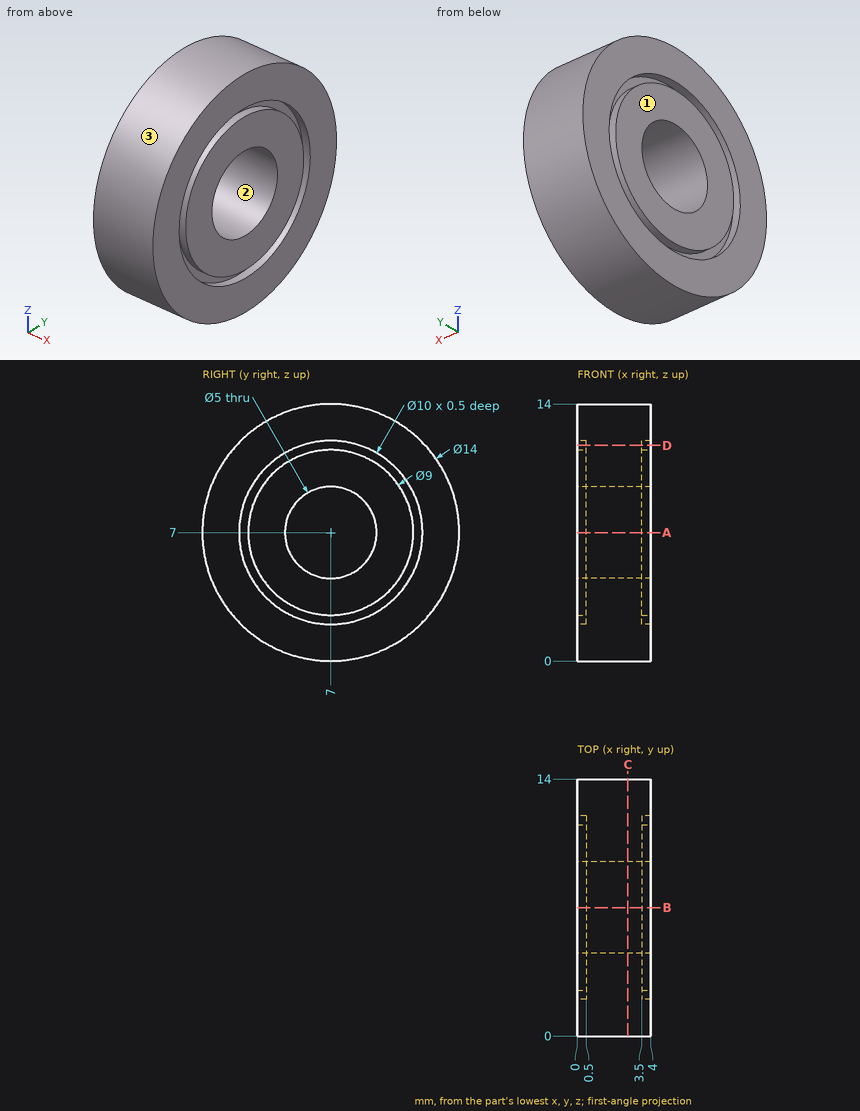
For this review, use the dimensioned drawing (mm, ordinates from the lowest corner) and the shaded views. Round coordinates to 2 decimals unless told otherwise and drop trailing zeros. Order: outer loops, then holes, each group sorted by start corner. A loop starts at its lowest first (then second) coordinate and runs counter-clockwise, first axis right, second up. Notation, with made-up numbers: (39, 10.5) -> (90, 10.5) arc R34 ccw to (90, 41.5) -> close; hole circle Ø4 at (62, 7.25). An arc over 180 degrees is marked (long way). One line per item, written item: value. Start each with the question number.
Q1. Clearance check with flat-ended pins moving along their axes: pin 1 Ø1 at (x, z) = (2, 3.5) entering from -Y; pin 2 Ø1 at (x, y) = (3, 12.5) entering from +Z. State where each tip first meets the part, or that it passes through.
Q2. Mouldability with a two-part tool opening along Z and no side actions: class the marked faces 1, 2 and 3 as released by +Z, released by -Z, zero draft, split by the parting line, or undercut.
Q3. Take a section at D-D (z = 11.75). Write out the cut boundary in (x, y), and give its area (3 significant figures).
Q4. Take a section at A-A (z = 7). Write out the cut boundary in (x, y).
Q5. Wall thickness on line 1 (Y direction, x = 3.65, z = 7); line 2 (Y direction, x = 3.55, z = 5.25); line 3 (Y direction, x = 0.6, z = 5): over which ranges is each line inside the solid? List them lowest first.
Q6. Take a section at C-C (x = 2.75). Write out the cut boundary in (y, z).
Reported:
1. pin 1: stops at y = 0.68
1. pin 2: stops at z = 11.9
2. face 1: zero draft
2. face 2: undercut
2. face 3: split by the parting line
3. outline: (0, 1.86) -> (4, 1.86) -> (4, 5.44) -> (3.5, 5.44) -> (3.5, 8.56) -> (4, 8.56) -> (4, 12.14) -> (0, 12.14) -> (0, 8.56) -> (0.5, 8.56) -> (0.5, 5.44) -> (0, 5.44) -> close
3. area: 38.0 mm2
4. outline: (0, 0) -> (4, 0) -> (4, 2) -> (3.5, 2) -> (3.5, 2.5) -> (4, 2.5) -> (4, 4.5) -> (0, 4.5) -> (0, 2.5) -> (0.5, 2.5) -> (0.5, 2) -> (0, 2) -> close; (0, 9.5) -> (4, 9.5) -> (4, 11.5) -> (3.5, 11.5) -> (3.5, 12) -> (4, 12) -> (4, 14) -> (0, 14) -> (0, 12) -> (0.5, 12) -> (0.5, 11.5) -> (0, 11.5) -> close
5. line 1: y = 0 to 2, 2.5 to 4.5, 9.5 to 11.5, 12 to 14
5. line 2: y = 0.22 to 2.32, 2.85 to 5.21, 8.79 to 11.15, 11.68 to 13.78
5. line 3: y = 0.29 to 5.5, 8.5 to 13.71
6. outline: circle Ø14 at (7, 7); hole circle Ø5 at (7, 7)
